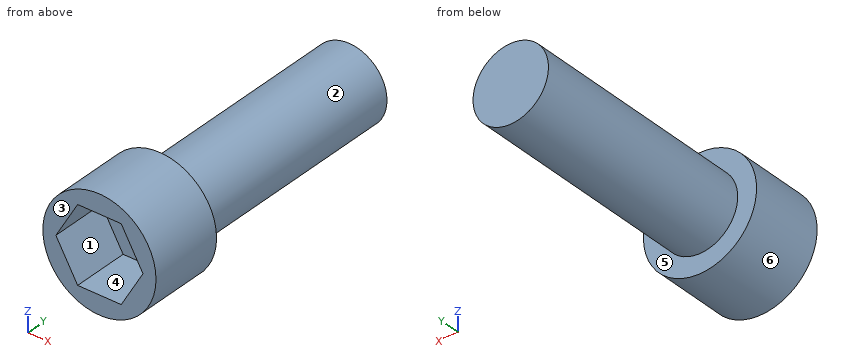
```python
from build123d import *

# Parameters (mm, degrees)
SKETCH1_R           = 4
BOSS_EXTRUDE1_DEPTH = 25
SKETCH2_R           = 6
SKETCH2_R_2         = 4
BOSS_EXTRUDE2_DEPTH = 2
SKETCH3_R           = 6
BOSS_EXTRUDE3_DEPTH = 6


with BuildPart() as part:
    # Sketch1 → Boss-Extrude1 (new body)
    with BuildSketch(Plane(origin=(0, 0, 0), x_dir=(1, 0, 0), z_dir=(0, 1, 0))):
        Circle(SKETCH1_R)
    extrude(amount=BOSS_EXTRUDE1_DEPTH)

    # Sketch2 → Boss-Extrude2 (add)
    with BuildSketch(Plane.XZ):
        Circle(SKETCH2_R)
        Circle(SKETCH2_R_2, mode=Mode.SUBTRACT)
        Circle(SKETCH2_R_2)
        Circle(SKETCH2_R_2)
    extrude(amount=BOSS_EXTRUDE2_DEPTH)

    # Sketch3 → Boss-Extrude3 (add)
    with BuildSketch(Plane.XZ.offset(2)):
        Circle(SKETCH3_R)
        Polygon((4.618802154, 0), (2.309401077, 4), (-2.309401077, 4), (-4.618802154, 0), (-2.309401077, -4), (2.309401077, -4), align=None, mode=Mode.SUBTRACT)
    extrude(amount=BOSS_EXTRUDE3_DEPTH)


solid = part.part
```
Design review of the part built by this model. Coordinates are the model's own, in mm. Face numbers are marked on the shaded views. A direction names the side the tool comes from. Round coordinates to 2 decimals unless told otherwise and drop trailing zeros. Order: outer loops, then holes, each group sorted by start corner. A loop starts at its lowest first (then second) coordinate and runs counter-clockwise, first axis right, second up. Notation, with made-up numbers: (44.5, 6) - (58.5, 6) arc R13 cw to (58.5, 20) - close; hole circle Ø10 at (44.5, 15). An arc over 180 degrees is marked (long way). Return JSON: item names as keys, results as strings.
Q1. For pin 1 Ø3 at (x, y) = (-1.5, 8.5) entering from +Z; pin 2 Ø5 at (y, z) = (7, 4.5) entering from +X; pin 3 Ø6 at (y, z) = (16.5, -4) entering from -X, all flat-tipped, find the tip position at first contact; note any pin that passes through.
Computed values:
{"pin 1": "stops at z = 4", "pin 2": "stops at x = 3.46", "pin 3": "stops at x = -3.87"}
Q2. Consider section B-B on x = 0. Write out the cut boundary in (y, z), plus the area to 3 significant figures.
Computed values:
{"outline": "(-8, -6) - (0, -6) - (0, -4) - (25, -4) - (25, 4) - (0, 4) - (0, 6) - (-8, 6) - (-8, 4) - (-2, 4) - (-2, -4) - (-8, -4) - close", "area": "248 mm2"}
Q3. Wall thickness on L1, parallel to Y at x = 0.5, z = -1; L2, parallel to Y at x = -2.5, z = 3.5; L3, parallel to Z at x = -5.25, y = -1.5: over which ranges is each line inside the solid? List them lowest first. Write a range as [from, to].
Computed values:
{"L1": "y = [-2, 25]", "L2": "y = [-2, 0]", "L3": "z = [-2.9, 2.9]"}
Q4. The part is to be moulded in two halves that separate along X. For the marked faces 4, 5 and 6, say which applies: pulls with the +X half, pulls with the -X half, needs draft (parallel to the pull), parting line crosses it, or undercut.
Computed values:
{"face 4": "undercut", "face 5": "needs draft", "face 6": "parting line crosses it"}
Q5. Consider section C-C on z = 1.75. Write out the cut boundary in (x, y).
Computed values:
{"outline": "(-5.74, -8) - (-3.61, -8) - (-3.61, -2) - (3.61, -2) - (3.61, -8) - (5.74, -8) - (5.74, 0) - (3.6, 0) - (3.6, 25) - (-3.6, 25) - (-3.6, 0) - (-5.74, 0) - close"}
Q6. Consider section D-D on y = 13. Write out the cut boundary in (x, z).
Computed values:
{"outline": "circle Ø8 at (0, 0)"}
Q7. Consider section A-A on y = -4.5. Write out the cut boundary in (x, z), plus the area to 3 significant figures.
Computed values:
{"outline": "circle Ø12 at (0, 0); hole (-4.62, 0) - (-2.31, -4) - (2.31, -4) - (4.62, 0) - (2.31, 4) - (-2.31, 4) - close", "area": "57.7 mm2"}
Q8. Machinability: for the marked faces 1, 2 and 3, which of the approach directions +Z, -Z, +X, -X, +Y, -Y give a long, thin tool a straight path to every point of the face, cutting with its end or side? Answer none if there is none.
Computed values:
{"face 1": "-Y", "face 2": "+Y", "face 3": "+Z, -Z, +X, -X, -Y"}
